CAD build for the part. Positions are in the model's coordinates, mm. Face numbers are marked on the shaded views. A direction names the side the tool comes from. Round coordinates to 2 decimals unless told otherwise and drop trailing zeros. Order: outer loops, then holes, each group sorted by start corner. A loop starts at its lowest first (then second) coordinate and runs counter-clockwise, first axis right, second up. Notation, with made-up numbers: (-18.5, -10.75) -> (31.5, -10.75) arc R26 cw to (31.5, 17.25) -> close; hole circle Ø7 at (-34.5, 22). An arc over 180 degrees is marked (long way). Return JSON: item names as keys, results as strings. Group by question number.
Q1. Cut at B-B (x = -20). Write the cut outline in (y, z) (3 decimals).
Q2. Probe line 1 along X through (y, z) = (-6.5, -4); line 2 along X through (y, z) = (3, 11); line 3 along Z through (x, y) = (-2.5, 0). List the from-to ranges inside material, lowest first.
Q3. Cut at A-A (x = -41). Count the separate pieces of the cut face and the enclosed holes in it, then the cut area to 3 significant figures.
Q4. Cut at C-C (x = -27). Write the cut outline in (y, z), then the cut area to 3 significant figures.
Q5. Flat gauge pins, fed straight in: pin 1 (2 mm diameter, centred on y = 7.5, z = -8, fed in from +X); pin 2 (4 mm diameter, centred on x = -30.5, y = -12.5, fed in from +Z); pin 3 (5.5 mm diameter, centred on y = 0, z = 0, fed in from -X). Where does each tip first touch, or does it go through?
Q6. Which spindle directions (+Z, -Z, +X, -X, +Y, -Y) get a long thin tool onto all of the face, cutting with end or side? Do the marked faces 1, 2 and 3. Say none if no direction does.
from build123d import *

# Parameters (mm, degrees)
COQUE1_START                 = -46
COQUE1_OUTLINE_R             = 14.9
COQUE1_DEPTH                 = 36
COQUE1_START_2               = -10
COQUE1_2_OUTLINE_R           = 10.5
COQUE1_2_DEPTH               = 2
COQUE1_START_3               = -34.9
COQUE1_3_OUTLINE_R           = 15
COQUE1_3_OUTLINE_R_2         = 14.9
COQUE1_3_DEPTH               = 17.8
COQUE1_START_4               = -47
COQUE1_4_OUTLINE_R           = 7
COQUE1_4_DEPTH               = 1
COQUE1_5_OUTLINE_R           = 15
COQUE1_5_OUTLINE_R_2         = 14.9
COQUE1_5_DEPTH               = 1
COQUE1_START_5               = -8
COQUE1_6_OUTLINE_R           = 0.5
COQUE1_6_DEPTH               = 3
CHANFREIN1_SIZE              = 0.5
ENL_V_MAT_EXTRU_1_REACH      = 62.959
ESQUISSE5_R                  = 3
R_P_TITION_CIRCULAIRE1_COUNT = 8
R_P_TITION_CIRCULAIRE2_COUNT = 6


# Read off the part's stored shape, not the designer's step: Coque1
with BuildPart() as part:
    # Esquisse1 → Base-Révolution (revolve)
    with BuildSketch(Plane.XY, mode=Mode.PRIVATE) as base_r_volution_sk:
        Polygon((-54, 5), (-54, 12), (-51, 12), (-51, 20), (-40, 20), (-40, 19.9), (-39.9, 19.9), (-39.9, 20), (-12.1, 20), (-12.1, 19.9), (-12, 19.9), (-12, 20), (-5, 20), (-5, 15.5), (-3, 15.5), (-3, 5.5), (0, 5.5), (0, 0), (-52, 0), (-52, 5), align=None)
    revolve(base_r_volution_sk.sketch.rotate(Axis((-92, 0, 0), (1, 0, 0)), 180), axis=Axis((-92, 0, 0), (1, 0, 0)))

    # Coque1 outline → Coque1 (cut)
    with BuildSketch(Plane.YZ.offset(COQUE1_START)):
        Circle(COQUE1_OUTLINE_R)
    extrude(amount=COQUE1_DEPTH, mode=Mode.SUBTRACT)

    # Coque1 2 outline → Coque1 2 (cut)
    with BuildSketch(Plane.YZ.offset(COQUE1_START_2)):
        Circle(COQUE1_2_OUTLINE_R)
    extrude(amount=COQUE1_2_DEPTH, mode=Mode.SUBTRACT)

    # Coque1 3 outline → Coque1 3 (cut)
    with BuildSketch(Plane.YZ.offset(COQUE1_START_3)):
        Circle(COQUE1_3_OUTLINE_R)
        Circle(COQUE1_3_OUTLINE_R_2, mode=Mode.SUBTRACT)
    extrude(amount=COQUE1_3_DEPTH, mode=Mode.SUBTRACT)

    # Coque1 4 outline → Coque1 4 (cut)
    with BuildSketch(Plane.YZ.offset(COQUE1_START_4)):
        Circle(COQUE1_4_OUTLINE_R)
    extrude(amount=COQUE1_4_DEPTH, mode=Mode.SUBTRACT)

    # Coque1 5 outline → Coque1 5 (cut)
    with BuildSketch(Plane.YZ.offset(COQUE1_START)):
        Circle(COQUE1_5_OUTLINE_R)
        Circle(COQUE1_5_OUTLINE_R_2, mode=Mode.SUBTRACT)
    extrude(amount=COQUE1_5_DEPTH, mode=Mode.SUBTRACT)

    # Coque1 6 outline → Coque1 6 (cut)
    with BuildSketch(Plane.YZ.offset(COQUE1_START_5)):
        Circle(COQUE1_6_OUTLINE_R)
    extrude(amount=COQUE1_6_DEPTH, mode=Mode.SUBTRACT)

    # Chanfrein1
    chanfrein1_edges = [part.edges().sort_by_distance(p)[0] for p in [
        (-54, 12, 0),
    ]]
    chamfer(chanfrein1_edges, length=CHANFREIN1_SIZE)

    # Esquisse5 → Enlèv. mat.-Extru.1 (cut, up to next)
    with BuildSketch(Plane(origin=(0, 0, 0), x_dir=(0, 0, -1), z_dir=(1, 0, 0)), mode=Mode.PRIVATE) as enl_v_mat_extru_1_sk1:
        with Locations(Location((0, 0, 0), (0, 0, 90))):
            Circle(ESQUISSE5_R)
    enl_v_mat_extru_1_tool1 = extrude(enl_v_mat_extru_1_sk1.sketch, amount=-ENL_V_MAT_EXTRU_1_REACH, mode=Mode.PRIVATE) & part.part
    add(enl_v_mat_extru_1_tool1.solids().sort_by_distance((0, 0, 0))[0], mode=Mode.SUBTRACT)

    # Esquisse4 → Trou taraudé M41 (revolve, cut)
    with BuildSketch(Plane(origin=(-51, 17.5, 0), x_dir=(0, 0, 1), z_dir=(0, 1, 0))):
        Polygon((0, 0), (0, 12.452627944), (1.65, 11.5), (1.65, 0), align=None)
    trou_taraud_m41 = revolve(axis=Axis((-57.35, 17.5, 0), (1, 0, 0)), mode=Mode.SUBTRACT)

    # Esquisse6 → Trou taraudé M2.51 (revolve, cut)
    with BuildSketch(Plane(origin=(-5, 17.5, 0), x_dir=(0, 0, -1), z_dir=(0, 1, 0))):
        Polygon((0, 0), (0, 20.591784026), (1.025, 20), (1.025, 0), align=None)
    trou_taraud_m2_51 = revolve(axis=Axis((1.35, 17.5, 0), (-1, 0, 0)), mode=Mode.SUBTRACT)

    # Répétition circulaire1: Trou taraudé M41 ×8 about axis
    r_p_tition_circulaire1_axis = Axis((0, 0, 0), (1, 0, 0))
    for i in range(1, R_P_TITION_CIRCULAIRE1_COUNT):
        add(trou_taraud_m41.rotate(r_p_tition_circulaire1_axis, i * 360 / R_P_TITION_CIRCULAIRE1_COUNT), mode=Mode.SUBTRACT)

    # Répétition circulaire2: Trou taraudé M2.51 ×6 about axis
    r_p_tition_circulaire2_axis = Axis((0, 0, 0), (1, 0, 0))
    for i in range(1, R_P_TITION_CIRCULAIRE2_COUNT):
        add(trou_taraud_m2_51.rotate(r_p_tition_circulaire2_axis, i * 360 / R_P_TITION_CIRCULAIRE2_COUNT), mode=Mode.SUBTRACT)


solid = part.part
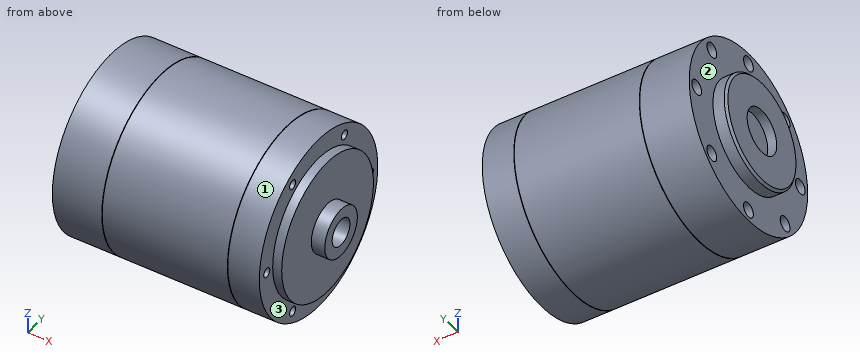
Solution:
{
 "1": {"outline": "circle Ø40 at (0, 0); hole circle Ø2.05 at (-17.5, 0); hole circle Ø30 at (0, 0); hole circle Ø2.05 at (-8.75, -15.155); hole circle Ø2.05 at (-8.75, 15.155); hole circle Ø2.05 at (8.75, -15.155); hole circle Ø2.05 at (8.75, 15.155); hole circle Ø2.05 at (17.5, 0)"},
 "2": {"line 1": "x = -54 to -46, -8 to -3", "line 2": "x = -54 to -46, -10 to -3", "line 3": "z = -5.5 to -3, 3 to 5.5"},
 "3": {"separate pieces": "1", "enclosed holes": "9", "area": "491 mm²"},
 "4": {"outline": "circle Ø40 at (0, 0); hole circle Ø30 at (0, 0)", "area": "550 mm²"},
 "5": {"pin 1": "stops at x = -3", "pin 2": "stops at z = 17.02", "pin 3": "stops at x = -52"},
 "6": {"face 1": "+X, -X", "face 2": "-X", "face 3": "+X"}
}
